For this review, use the dimensioned drawing (mm, ordinates from the lowest corner) and the shaded views. Coordinates: 2 decimals unless noted, no trailing zeros. Order: outer loops, then holes, each group sorted by start corner. A loop starts at its lowest first (then second) coordinate and runs counter-clockwise, first axis right, second up. Notation, with made-up numbers: (-12, -30) -> (15, -30) arc R10 cw to (15, -26) -> close; hole circle Ø1 at (63.25, 30.5). An arc over 180 degrees is marked (long way). Return JSON: item names as keys, results as strings. Group by question number.
Item 1: Draft analysis for pull direction Z (two halves, no side actions). For the marked faces 1, 2 and 3, state which applies: +Z half, -Z half, draft (parallel to the pull), parting line (faces both ways), or undercut.
Item 2: Take a section at C-C (x = 39). Write out the cut boundary in (y, z), then the cut area to 3 significant figures.
Item 3: For line 1 along Y through (x, z) = (20.5, 12.5); line 2 along Y through (x, z) = (38, 5); line 3 along Y through (x, z) = (7, 2.5), list the stretches that pass through material, from the lowest coordinate up.
Item 4: Take a section at B-B (y = 52.5). Write out the cut boundary in (x, z), then the cut area to 3 significant figures.
Item 5: Take a section at D-D (x = 7). Write out the cut boundary in (y, z), then the cut area to 3 significant figures.
Item 6: Insertion check: pin 1 (6.5 mm diameter, centred on x = 7, y = 64, fed in from +Z); pin 2 (2.5 mm diameter, centred on y = 63.5, z = 4, fed in from +X); pin 3 (3 mm diameter, centred on x = 7, y = 17.5, fed in from -Z). Each pin has a flat end and moves straight along its axis. Give the tip position at first contact, or say it passes through.
Item 7: Take a section at A-A (z = 12.5). Count the separate pieces of the cut face and the enclosed holes in it, then the cut area to 3 significant figures.
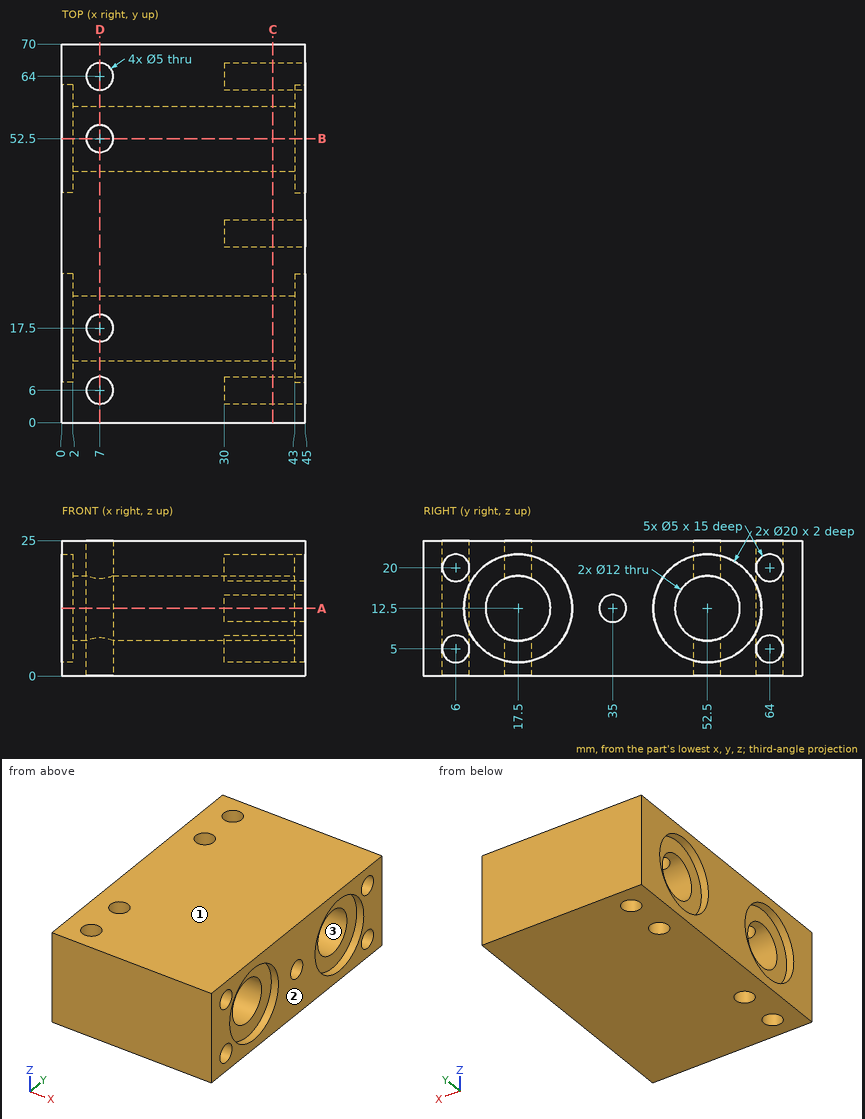
Findings below:
{
 "1": {"face 1": "+Z half", "face 2": "draft", "face 3": "undercut"},
 "2": {"outline": "(0, 0) -> (70, 0) -> (70, 25) -> (0, 25) -> close; hole circle Ø5 at (6, 5); hole circle Ø5 at (6, 20); hole circle Ø12 at (17.5, 12.5); hole circle Ø5 at (35, 12.5); hole circle Ø12 at (52.5, 12.5); hole circle Ø5 at (64, 5); hole circle Ø5 at (64, 20)", "area": "1,430 mm2"},
 "3": {"line 1": "y = 0 to 11.5, 23.5 to 46.5, 58.5 to 70", "line 2": "y = 0 to 3.5, 8.5 to 61.5, 66.5 to 70", "line 3": "y = 0 to 3.5, 8.5 to 15, 20 to 50, 55 to 61.5, 66.5 to 70"},
 "4": {"outline": "(0, 0) -> (4.5, 0) -> (4.5, 6.5) -> (2, 6.5) -> (2, 2.5) -> (0, 2.5) -> close; (0, 22.5) -> (2, 22.5) -> (2, 18.5) -> (4.5, 18.5) -> (4.5, 25) -> (0, 25) -> close; (9.5, 0) -> (45, 0) -> (45, 2.5) -> (43, 2.5) -> (43, 6.5) -> (9.5, 6.5) -> close; (9.5, 18.5) -> (43, 18.5) -> (43, 22.5) -> (45, 22.5) -> (45, 25) -> (9.5, 25) -> close", "area": "488 mm2"},
 "5": {"outline": "(0, 0) -> (3.5, 0) -> (3.5, 25) -> (0, 25) -> close; (8.5, 0) -> (15, 0) -> (15, 7.05) arc R6 cw to (15, 17.95) -> (15, 25) -> (8.5, 25) -> close; (20, 0) -> (50, 0) -> (50, 7.05) arc R6 cw to (50, 17.95) -> (50, 25) -> (20, 25) -> (20, 17.95) arc R6 cw to (20, 7.05) -> close; (55, 0) -> (61.5, 0) -> (61.5, 25) -> (55, 25) -> (55, 17.95) arc R6 cw to (55, 7.05) -> close; (66.5, 0) -> (70, 0) -> (70, 25) -> (66.5, 25) -> close", "area": "1,140 mm2"},
 "6": {"pin 1": "stops at z = 25", "pin 2": "stops at x = 30", "pin 3": "passes through"},
 "7": {"separate pieces": "3", "enclosed holes": "2", "area": "1,890 mm2"}
}
